Here's how the part is built. I have some questions about the finished solid (model axes, mm). A direction names the side the tool comes from. Round coordinates to 2 decimals unless told otherwise and drop trailing zeros. Loops run counter-clockwise (first coordinate to the right, second up) from the corner with the lowest first, then second, coordinate; pieces in that order, holes last. Notation, with made-up numbers: M 1.25,42 L 39.25,42 A10 ccw 39.25,50 Z; hole C -21.75,75 d8. An arc over 180 degrees is marked long. Answer as a JSON object with one key per item and string values.
from build123d import *

# Parameters (mm, degrees)
F0_W     = 152.4
F0_H     = 152.4
F1_DEPTH = 152.4
F2_W     = 12.7
F2_H     = 12.7
F3_DEPTH = 63.5
F4_DEPTH = 149.86


with BuildPart() as f1:
    # F0 (on Front) → F1 (new body)
    with BuildSketch(Plane.XZ):
        with Locations((-76.2, 76.2)):
            Rectangle(F0_W, F0_H)
    extrude(amount=F1_DEPTH)

    # F2 (on face) → F3 (join)
    with BuildSketch(Plane.XZ.offset(152.4)):
        with Locations((-6.35, 6.35)):
            Rectangle(F2_W, F2_H)
        with Locations((-107.95, 6.35)):
            Rectangle(F2_W, F2_H)
        with Locations((-107.95, 133.35)):
            Rectangle(F2_W, F2_H)
        with Locations((-44.45, 69.85)):
            Rectangle(F2_W, F2_H)
        with Locations((-107.95, 57.15)):
            Rectangle(F2_W, F2_H)
        with Locations((-44.45, 146.05)):
            Rectangle(F2_W, F2_H)
        with Locations((-146.05, 95.25)):
            Rectangle(F2_W, F2_H)
        with Locations((-82.55, 69.85)):
            Rectangle(F2_W, F2_H)
    extrude(amount=F3_DEPTH)

    # F0 (on Front) → F4 (cut)
    with BuildSketch(Plane.XZ):
        with Locations((-76.2, 76.2)):
            Rectangle(F0_W, F0_H)
    extrude(amount=F4_DEPTH, mode=Mode.SUBTRACT)


solid = f1.part
Item 1: I want a section at C-C on z = 95. List the corners of the cut face in (x, y) for me, plus the area to 3 significant figures.
Solution:
{"outline": "M -152.4,-215.9 L -139.7,-215.9 L -139.7,-152.4 L 0,-152.4 L 0,-149.86 L -152.4,-149.86 Z", "area": "1,190 mm2"}
Item 2: If I drill on L1, parallel to X at y = -212.5, z = 72; L2, parallel to Y at x = -25.5, z = 55; L3, parallel to X at y = -182.5, z = 95, over which ranges is the centre line in solid material (lowest first)? Write a range as from..to.
Solution:
{"L1": "x = -88.9..-76.2, -50.8..-38.1", "L2": "y = -152.4..-149.86", "L3": "x = -152.4..-139.7"}
Item 3: I want a section at D-D on x = -46.5. List the corners of the cut face in (y, z) for me, plus the area to 3 significant figures.
Solution:
{"outline": "M -215.9,63.5 L -152.4,63.5 L -152.4,0 L -149.86,0 L -149.86,152.4 L -215.9,152.4 L -215.9,139.7 L -152.4,139.7 L -152.4,76.2 L -215.9,76.2 Z", "area": "2,000 mm2"}
Item 4: We'd pull the mould along X, two halves only. Please class faces 1 (the face through (-38.1, -184, 146)), 2 (the face through (-101.6, -184, 6)), 3 (the face through (-50.8, -184, 70)), 4 (the face through (-114.3, -184, 57)): +X half, -X half, draft (parallel to the pull), parting line (faces both ways), or undercut.
Solution:
{"face 1": "+X half", "face 2": "undercut", "face 3": "undercut", "face 4": "-X half"}
Item 5: I want a section at B-B on x = -111.5. List the corners of the cut face in (y, z) for me.
Solution:
{"outline": "M -215.9,0 L -149.86,0 L -149.86,152.4 L -152.4,152.4 L -152.4,139.7 L -215.9,139.7 L -215.9,127 L -152.4,127 L -152.4,63.5 L -215.9,63.5 L -215.9,50.8 L -152.4,50.8 L -152.4,12.7 L -215.9,12.7 Z"}
Item 6: I want a section at A-A on y = -167. Count the separate pieces of the cut face and the enclosed holes in it, plus the area to 3 significant figures.
Solution:
{"separate pieces": "8", "enclosed holes": "0", "area": "1,290 mm2"}
Item 7: For faces 5 (the face through (-108, -184, 139.7)), 6 (the face through (-108, -184, 127)), 7 (the face through (-114.3, -184, 6)), 8 (the face through (-101.6, -184, 57)), 9 (the face through (-6, -184, 12.7)), which set-ups out of +Z, -Z, +X, -X, +Y, -Y let a thin tool reach every point of the face, with its end or its side?
Solution:
{"face 5": "+Z, -X, -Y", "face 6": "+X, -X, -Y", "face 7": "+Z, -Z, -X, -Y", "face 8": "+Z, -Z, +X, -Y", "face 9": "+Z, +X, -X, -Y"}
Item 8: For P1, Ø8, axis at x = -42, y = -209, coming from the -Z side; P2, Ø14, axis at x = -108, y = -194, coming from the +Z side; P3, Ø10, axis at y = -175, z = 96, coming from the +X side, each with a flat end and sliding along its axis, tell me the tip position at first contact or that it passes through.
Solution:
{"P1": "stops at z = 63.5", "P2": "stops at z = 139.7", "P3": "stops at x = -139.7"}
